Here's how the part is built. I have some questions about the finished solid (model axes, mm). Coordinates: 2 decimals unless noted, no trailing zeros. Loops run counter-clockwise (first coordinate to the right, second up) from the corner with the lowest first, then second, coordinate; pieces in that order, holes last. Notation, with made-up numbers: M 44.5,-31.75 L 82.5,-31.75 A8 cw 82.5,-24.75 Z; hole C 75,57 d4. An arc over 180 degrees is marked long. Use one line per item in the form item = value. Start each with the question number.
(1) Will this pin go through, and if not, where does the flat tip stop? P1, Ø1.5, axis at x = -300.5, y = 48.5, coming from the -Z side.
(2) Imagine slicing it at C-C, the plane z = 2. State how many separate pieces and enclosed holes the cut face has, and give its area (3 significant figures).
(3) Imagine slicing it at A-A, the plane y = 41. Please give me the cut outline in (x, z).
(4) Imagine slicing it at B-B, the plane x = -396.5. Please give me the cut outline in (y, z).
(5) Please list where these lines run through material, in increasing order: L1, parallel to X at y = 59, z = 0.85; L2, parallel to X at y = 125, z = 0.75; L3, parallel to Y at x = -340.5, z = 2.3.
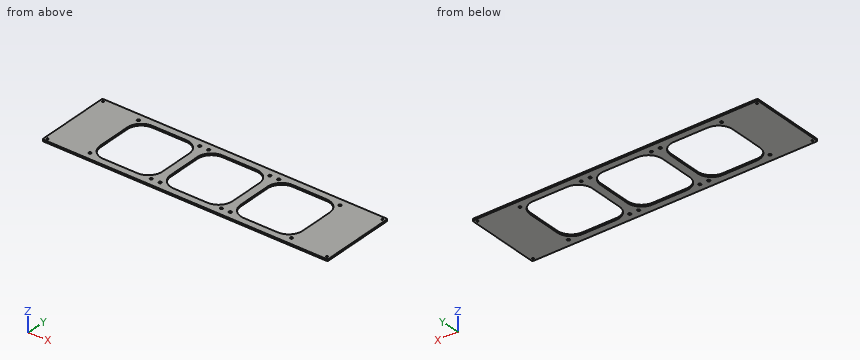
Autodesk Inventor part; units mm, degrees
ref_plane "YZ Plane" through (0, 0, 0) normal (1, 0, 0) x (0, 1, 0)
ref_plane "XZ Plane" through (0, 0, 0) normal (0, 1, 0) x (-1, 0, 0)
ref_plane "XY Plane" through (0, 0, 0) normal (0, 0, 1) x (1, 0, 0)
sketch "スケッチ1" plane through (0, 0, 0) normal (0, 0, 1) x (1, 0, 0)
  circle A0 centre (5, 125) radius 2.25 construction
  circle A1 centre (5, 5) radius 2.25 construction
  circle A2 centre (-473, 125) radius 2.25 construction
  circle A3 centre (-473, 5) radius 2.25 construction
  line L0 (-478, 130) -> (-478, 0) construction
  line L1 (10, 0) -> (10, 130) construction
  line L2 (10, 130) -> (-478, 130)
  line L3 (-478, 130) -> (-478, 0)
  line L4 (-478, 0) -> (10, 0)
  line L5 (10, 0) -> (10, 130)
  circle A4 centre (5, 125) radius 1.6
  circle A5 centre (5, 5) radius 1.6
  circle A6 centre (-473, 5) radius 1.6
  circle A7 centre (-473, 125) radius 1.6
  line L6 (10, 65) -> (-478, 65) construction
  line L7 (-205, 118) -> (-263, 118)
  line L8 (-287, 94) -> (-287, 36)
  line L9 (-263, 12) -> (-205, 12)
  line L10 (-181, 36) -> (-181, 94)
  arc A8 (-181, 94) -> (-205, 118) centre (-205, 94) ccw
  arc A9 (-205, 12) -> (-181, 36) centre (-205, 36) ccw
  arc A10 (-287, 36) -> (-263, 12) centre (-263, 36) ccw
  arc A11 (-263, 118) -> (-287, 94) centre (-263, 94) ccw
  line L11 (-174, 125) -> (-294, 125) construction
  line L12 (-294, 125) -> (-294, 5) construction
  line L13 (-294, 5) -> (-174, 5) construction
  line L14 (-174, 5) -> (-174, 125) construction
  line L15 (-181.6, 117.4) -> (-286.4, 117.4) construction
  line L16 (-286.4, 117.4) -> (-286.4, 12.6) construction
  line L17 (-286.4, 12.6) -> (-181.6, 12.6) construction
  line L18 (-181.6, 12.6) -> (-181.6, 117.4) construction
  circle A12 centre (-181.6, 117.4) radius 2.25
  circle A13 centre (-181.6, 12.6) radius 2.25
  circle A14 centre (-286.4, 12.6) radius 2.25
  circle A15 centre (-286.4, 117.4) radius 2.25
  circle A16 centre (-301.6, 117.4) radius 2.25
  arc A17 (-301, 94) -> (-325, 118) centre (-325, 94) ccw
  line L19 (-301, 36) -> (-301, 94)
  arc A18 (-325, 12) -> (-301, 36) centre (-325, 36) ccw
  circle A19 centre (-301.6, 12.6) radius 2.25
  line L20 (-383, 12) -> (-325, 12)
  arc A20 (-407, 36) -> (-383, 12) centre (-383, 36) ccw
  circle A21 centre (-406.4, 12.6) radius 2.25
  line L21 (-407, 94) -> (-407, 36)
  circle A22 centre (-406.4, 117.4) radius 2.25
  arc A23 (-383, 118) -> (-407, 94) centre (-383, 94) ccw
  line L22 (-325, 118) -> (-383, 118)
  circle A24 centre (-61.6, 117.4) radius 2.25
  arc A25 (-61, 94) -> (-85, 118) centre (-85, 94) ccw
  line L23 (-61, 36) -> (-61, 94)
  arc A26 (-85, 12) -> (-61, 36) centre (-85, 36) ccw
  circle A27 centre (-61.6, 12.6) radius 2.25
  line L24 (-143, 12) -> (-85, 12)
  arc A28 (-167, 36) -> (-143, 12) centre (-143, 36) ccw
  circle A29 centre (-166.4, 12.6) radius 2.25
  line L25 (-167, 94) -> (-167, 36)
  circle A30 centre (-166.4, 117.4) radius 2.25
  arc A31 (-143, 118) -> (-167, 94) centre (-143, 94) ccw
  line L26 (-85, 118) -> (-143, 118)
  circle A32 centre (-181.6, 117.4) radius 2.25
  arc A33 (-181, 94) -> (-205, 118) centre (-205, 94) ccw
  line L27 (-181, 36) -> (-181, 94)
  arc A34 (-205, 12) -> (-181, 36) centre (-205, 36) ccw
  circle A35 centre (-181.6, 12.6) radius 2.25
  line L28 (-263, 12) -> (-205, 12)
  arc A36 (-287, 36) -> (-263, 12) centre (-263, 36) ccw
  circle A37 centre (-286.4, 12.6) radius 2.25
  line L29 (-287, 94) -> (-287, 36)
  circle A38 centre (-286.4, 117.4) radius 2.25
  arc A39 (-263, 118) -> (-287, 94) centre (-263, 94) ccw
  line L30 (-205, 118) -> (-263, 118)
  point P0 (0, 0)
  point P1 (-234, 65)
  point P2 (-287, 12)
  point P3 (-287, 118)
  point P4 (-181, 12)
  point P5 (-287, 65)
  point P6 (-294, 65)
  point P7 (-234, 12)
  point P8 (-234, 5)
  point P9 (-234, 118)
  point P10 (-181, 65)
  point P11 (-174, 65)
  point P12 (-181.6, 65)
  point P13 (-234, 125)
  point P14 (-234, 117.4)
  point P15 (-301, 12)
  point P16 (-301, 65)
  point P17 (-407, 12)
  point P18 (-354, 12)
  point P19 (-407, 118)
  point P20 (-407, 65)
  point P21 (-354, 118)
  point P22 (-61, 12)
  point P23 (-61, 65)
  point P24 (-167, 12)
  point P25 (-114, 12)
  point P26 (-167, 118)
  point P27 (-167, 65)
  point P28 (-114, 118)
  point P29 (-181, 12)
  point P30 (-181, 65)
  point P31 (-287, 12)
  point P32 (-234, 12)
  point P33 (-287, 118)
  point P34 (-287, 65)
  point P35 (-234, 118)
  dimension "d0" = 3.2
  dimension "d1" = 106
  dimension "d2" = 106
  dimension "d3" = 24
  dimension "d4" = 120
  dimension "d5" = 120
  dimension "d6" = 104.8
  dimension "d7" = 104.8
  dimension "d8" = 4.5
  dimension "d11" = 120
  dimension "d14" = 120
extrude "押し出し1" add sketch "スケッチ1" along normal blind 3
sketch "スケッチ2" plane through (0, 0, 3) normal (0, 0, 1) x (1, 0, 0)
  line L0 (-478, 130) -> (-478, 0)
  line L1 (-478, 0) -> (10, 0)
  line L2 (10, 0) -> (10, 130)
  line L3 (10, 130) -> (-478, 130)
  circle A0 centre (-286.4, 117.4) radius 2.25
  arc A1 (-263, 118) -> (-287, 94) centre (-263, 94) ccw
  line L4 (-263, 118) -> (-205, 118)
  arc A2 (-181, 94) -> (-205, 118) centre (-205, 94) ccw
  line L5 (-181, 94) -> (-181, 36)
  arc A3 (-205, 12) -> (-181, 36) centre (-205, 36) ccw
  line L6 (-205, 12) -> (-263, 12)
  arc A4 (-287, 36) -> (-263, 12) centre (-263, 36) ccw
  line L7 (-287, 36) -> (-287, 94)
  circle A5 centre (-473, 125) radius 1.6
  circle A6 centre (-473, 5) radius 1.6
  circle A7 centre (5, 5) radius 1.6
  circle A8 centre (5, 125) radius 1.6
  circle A9 centre (-181.6, 117.4) radius 2.25
  circle A10 centre (-181.6, 12.6) radius 2.25
  circle A11 centre (-286.4, 12.6) radius 2.25
  circle A12 centre (-166.4, 117.4) radius 2.25
  circle A13 centre (-166.4, 12.6) radius 2.25
  circle A14 centre (-61.6, 12.6) radius 2.25
  line L8 (-61, 94) -> (-61, 36)
  arc A15 (-85, 12) -> (-61, 36) centre (-85, 36) ccw
  line L9 (-85, 12) -> (-143, 12)
  arc A16 (-167, 36) -> (-143, 12) centre (-143, 36) ccw
  line L10 (-167, 36) -> (-167, 94)
  arc A17 (-143, 118) -> (-167, 94) centre (-143, 94) ccw
  line L11 (-143, 118) -> (-85, 118)
  arc A18 (-61, 94) -> (-85, 118) centre (-85, 94) ccw
  circle A19 centre (-61.6, 117.4) radius 2.25
  circle A20 centre (-406.4, 117.4) radius 2.25
  circle A21 centre (-406.4, 12.6) radius 2.25
  circle A22 centre (-301.6, 12.6) radius 2.25
  line L12 (-301, 94) -> (-301, 36)
  arc A23 (-325, 12) -> (-301, 36) centre (-325, 36) ccw
  line L13 (-325, 12) -> (-383, 12)
  arc A24 (-407, 36) -> (-383, 12) centre (-383, 36) ccw
  line L14 (-407, 36) -> (-407, 94)
  arc A25 (-383, 118) -> (-407, 94) centre (-383, 94) ccw
  line L15 (-383, 118) -> (-325, 118)
  arc A26 (-301, 94) -> (-325, 118) centre (-325, 94) ccw
  circle A27 centre (-301.6, 117.4) radius 2.25
  line L16 (-477.9, 129.9) -> (-477.9, 0.1)
  line L17 (-477.9, 0.1) -> (9.9, 0.1)
  line L18 (9.9, 0.1) -> (9.9, 129.9)
  line L19 (9.9, 129.9) -> (-477.9, 129.9)
  point P0 (0, 0)
  dimension "d19" = 0.1
extrude "押し出し2" cut sketch "スケッチ2" against normal through all contours L3 L2 L1 L0
fillet "フィレット1" radius 2 4 edges at (-477.9, 129.9, 1.5) (-477.9, 0.1, 1.5) (9.9, 0.1, 1.5) (9.9, 129.9, 1.5)
equation "\"d5\" = d4"
equation "\"d7\" = d6"
properties part number "radiator_adapter_03"
Answer:
q1.P1 = 0
q2.separate_pieces = 1
q2.enclosed_holes = 19
q2.area = 30,900 mm²
q3.outline = M -477.9,0 L -407,0 L -407,3 L -477.9,3 Z; M -301,0 L -287,0 L -287,3 L -301,3 Z; M -181,0 L -167,0 L -167,3 L -181,3 Z; M -61,0 L 9.9,0 L 9.9,3 L -61,3 Z
q4.outline = M 0.1,0 L 16.16,0 L 16.16,3 L 0.1,3 Z; M 113.84,0 L 129.9,0 L 129.9,3 L 113.84,3 Z
q5.L1 = -477.9 to -407, -301 to -287, -181 to -167, -61 to 9.9
q5.L2 = -477.9 to -474.6, -471.4 to 3.4, 6.6 to 9.9
q5.L3 = 0.1 to 12, 118 to 129.9
